Work out the finished part from the listing and answer in its coordinate system (mm). A direction names the side the tool comes from. Round coordinates to 2 decimals unless told otherwise and drop trailing zeros. Loops run counter-clockwise (first coordinate to the right, second up) from the corner with the lowest first, then second, coordinate; pieces in that order, holes last. Notation, with made-up numbers: (9.25, 21.5) - (67.25, 21.5) arc R24 cw to (67.25, 53.5) - close; hole circle Ø9 at (-29.75, -13). An arc over 180 degrees is marked (long way). Answer as CSV lines item,"result". Start each with the question number.
Q1. Straight lines are drawn through the part: L1, parallel to Y at x = 2, z = -26; L2, parallel to Y at x = -34.5, z = -25.5; L3, parallel to X at y = 12.5, z = 10.5. For each, find the intervals that lie inside material, in ascending order. Write a range as [from, to].
Q2. Section A-A on z = 0 is taken. Write down the section's boundary in (x, y).
Q3. For faces 1 (the face through (-2.17, -8.38, 9.76)), 2 (the face through (0, -17, 0)), determine the directions among +Z, -Z, +X, -X, +Y, -Y from which every point of the face is accessible in a straight line to the end or side of a thin tool.
Q4. Section D-D on y = 12.5 is taken. Write down the section's boundary in (x, z).
Q5. Each of these flat-tipped pins is pushed along its axis until it touches: pin 1 Ø2 at (y, z) = (11.5, 28) entering from +X; pin 2 Ø8 at (x, y) = (-4.5, 14.5) entering from -Z; pin 3 Ø6 at (x, z) = (0, -32.5) entering from -Y. Where does it stop, or does it pass through?
Q6. Section C-C on y = -5.5 is taken. Write down the section's boundary in (x, z).
Q7. Section B-B on x = 0 is taken. Write down the section's boundary in (y, z), then the cut area to 3 significant figures.
Autodesk Inventor part; units mm, degrees
ref_plane "YZ Plane" through (0, 0, 0) normal (1, 0, 0) x (0, 1, 0)
ref_plane "XZ Plane" through (0, 0, 0) normal (0, 1, 0) x (-1, 0, 0)
ref_plane "XY Plane" through (0, 0, 0) normal (0, 0, 1) x (1, 0, 0)
sketch "Sketch1" plane through (0, 0, 0) normal (0, 1, 0) x (-1, 0, 0)
  circle A0 centre (0, 0) radius 47.15
  dimension "d0" = 94.3
extrude "Extrusion1" add sketch "Sketch1" along normal blind 25.4
fillet "Fillet1" radius 10 1 edges at (47.15, 25.4, 0)
sketch "Sketch2" plane through (0, 0, 0) normal (0, -1, 0) x (1, 0, 0)
  circle A0 centre (0, 0) radius 10
  dimension "d4" = 20
extrude "Extrusion2" add sketch "Sketch2" along normal blind 17
thread "Thread1"
properties part number "A.80.A.101111"
Findings:
1,L1,"y = [0, 25.4]"
1,L2,"y = [0, 23.58]"
1,L3,"x = [-45.97, 45.97]"
2,outline,"(-47.15, 0) - (-10, 0) - (-10, -17) - (10, -17) - (10, 0) - (47.15, 0) - (47.15, 15.4) arc R10 ccw to (37.15, 25.4) - (-37.15, 25.4) arc R10 ccw to (-47.15, 15.4) - close"
3,face 1,"-Y"
3,face 2,"+Z, -Z, +X, -X, -Y"
4,outline,"circle Ø94.3 at (0, 0)"
5,pin 1,"stops at x = 38.65"
5,pin 2,"stops at z = -47.15"
5,pin 3,"stops at y = 0"
6,outline,"circle Ø20 at (0, 0)"
7,outline,"(-17, -10) - (0, -10) - (0, -47.15) - (15.4, -47.15) arc R10 ccw to (25.4, -37.15) - (25.4, 37.15) arc R10 ccw to (15.4, 47.15) - (0, 47.15) - (0, 10) - (-17, 10) - close"
7,area,"2,690 mm^2"
